Design review of the part shown in the three views and the two pictorial views. Dimensions are in mm from the part's minimum x, y and z. A direction names the side the tool comes from. Coordinates: 2 decimals unless noted, no trailing zeros. Write each loop counter-clockwise with the first axis right and the second up, starting at its lowest first coordinate (ties: lowest second). Pieces come first, ordered by that corner, then holes.
Q1. For L1, parallel to Z at x = 11.5, y = 18.5 (1 decimal); L2, parallel to Z at x = 11, y = 19 (1 decimal); L3, parallel to Z at x = 12.7, y = 6.5, list the stretches that pass through material, from the lowest coordinate up.
Q2. Take a section at A-A, the plane x = 12.7. State how many separate pieces and enclosed holes the cut face has, plus the area to 3 significant figures.
Q3. For the marked faces 1, 2 and 3, list the 3-axis set-ups (+Z, -Z, +X, -X, +Y, -Y) from which the entire face can be reached by the end or side of a thin tool; tool diameter is ignored.
Q4. Take a section at D-D, the plane z = 18. Write out the cut boundary in (x, y) (1 decimal), plus the area to 3 significant figures.
Q5. For pin 1 Ø2.5 at (x, z) = (12.7, 22.225) entering from -Y; pin 2 Ø8 at (y, z) = (8.5, 14.5) entering from -X; pin 3 Ø2 at (x, y) = (13, 5.5) entering from -Z; pin 4 Ø5 at (x, z) = (12.5, 8.5) entering from +Y, all flat-tipped, find the tip position at first contact; note any pin that passes through.
Q6. The part is to be moulded in two halves that separate along X. For the marked faces 4, 5 and 6, say which applies: released by +X, released by -X, zero draft, split by the parting line, or undercut.
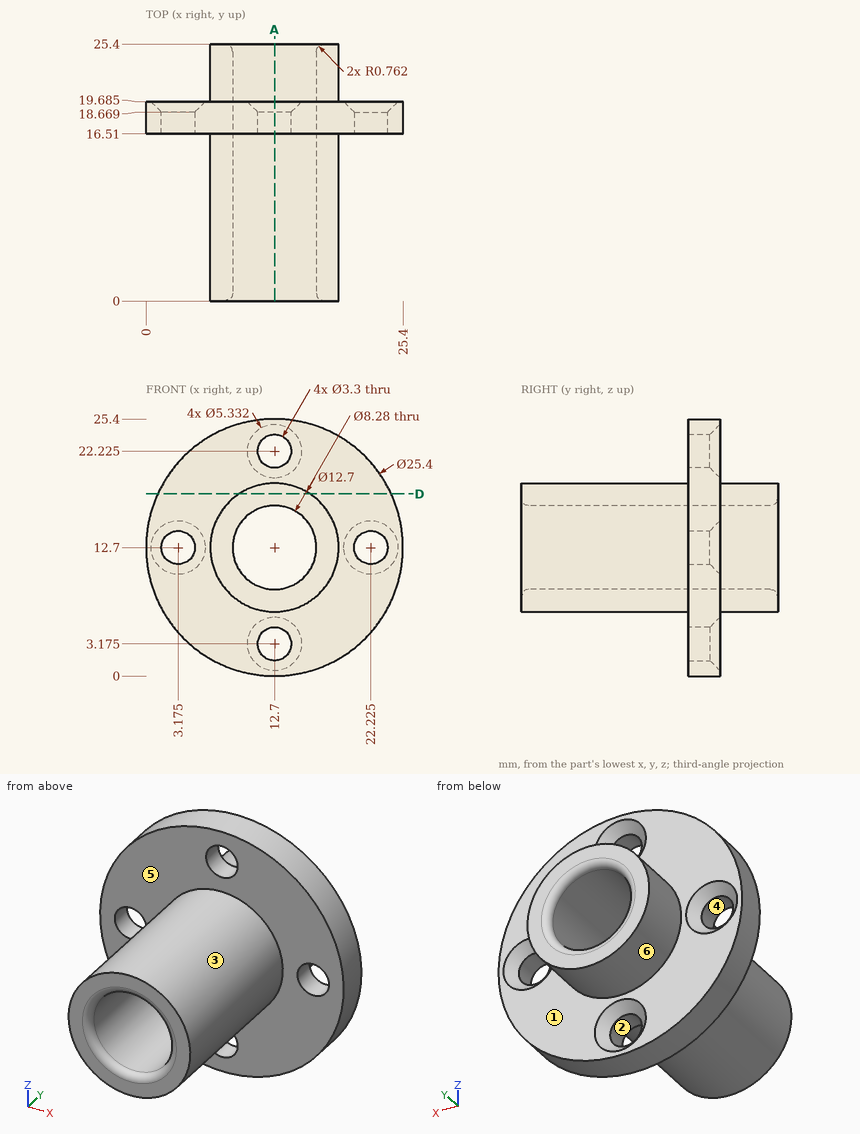
Responses:
1. L1: z = 0.1 to 2, 4.3 to 8.7, 16.7 to 21.1, 23.4 to 25.3
1. L2: z = 0.1 to 2.2, 4.2 to 8.9, 16.5 to 21.2, 23.2 to 25.3
1. L3: z = 6.35 to 8.56, 16.84 to 19.05
2. separate pieces: 4
2. enclosed holes: 0
2. area: 129 mm2
3. face 1: +Y
3. face 2: +Y, -Y
3. face 3: -Y
4. outline: (1.2, 16.5) - (9.2, 16.5) - (9.2, 0) - (16.2, 0) - (16.2, 16.5) - (24.2, 16.5) - (24.2, 19.7) - (16.2, 19.7) - (16.2, 25.4) - (9.2, 25.4) - (9.2, 19.7) - (1.2, 19.7) - close
4. area: 229 mm2
5. pin 1: passes through
5. pin 2: stops at x = 6.35
5. pin 3: stops at z = 6.35
5. pin 4: stops at y = 25.4
6. face 4: undercut
6. face 5: zero draft
6. face 6: split by the parting line
